from build123d import *

# Parameters (mm, degrees)
BOSS_EXTRUDE1_DEPTH = 1


with BuildPart() as part:
    # Sketch2 → Boss-Extrude1 (new body)
    with BuildSketch(Plane(origin=(0, 0, 0), x_dir=(1, 0, 0), z_dir=(0, 1, 0))):
        with BuildLine():
            Line((-6, 1), (-1, 1))
            Line((-1, 1), (-1, 6))
            ThreePointArc((-1, 6), (-0.853553391, 6.353553391), (-0.5, 6.5))
            Line((-0.5, 6.5), (0.5, 6.5))
            ThreePointArc((0.5, 6.5), (0.853553391, 6.353553391), (1, 6))
            Line((1, 6), (1, 1))
            Line((1, 1), (6, 1))
            ThreePointArc((6, 1), (6.353553391, 0.853553391), (6.5, 0.5))
            Line((6.5, 0.5), (6.5, -0.5))
            ThreePointArc((6.5, -0.5), (6.353553391, -0.853553391), (6, -1))
            Line((6, -1), (1, -1))
            Line((1, -1), (1, -6))
            ThreePointArc((1, -6), (0.853553391, -6.353553391), (0.5, -6.5))
            Line((0.5, -6.5), (-0.5, -6.5))
            ThreePointArc((-0.5, -6.5), (-0.853553391, -6.353553391), (-1, -6))
            Line((-1, -6), (-1, -1))
            Line((-1, -1), (-6, -1))
            ThreePointArc((-6, -1), (-6.353553391, -0.853553391), (-6.5, -0.5))
            Line((-6.5, -0.5), (-6.5, 0.5))
            ThreePointArc((-6.5, 0.5), (-6.353553391, 0.853553391), (-6, 1))
        make_face()
    extrude(amount=BOSS_EXTRUDE1_DEPTH)


solid = part.part
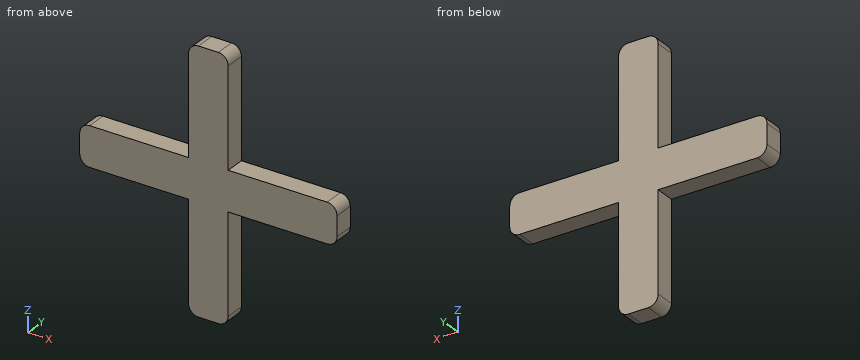
Geometry check sheet. Reference: the model listing, model coordinates, mm. Round coordinates to 2 decimals unless told otherwise and drop trailing zeros. Loops run counter-clockwise (first coordinate to the right, second up) from the corner with the lowest first, then second, coordinate; pieces in that order, holes last. Notation, with made-up numbers: (-38, 88.5) -> (13, 88.5) arc R20 cw to (13, 110.5) -> close; hole circle Ø4 at (11, 18). An arc over 180 degrees is marked (long way). Answer as a JSON object with one key per item and string values. Group by question number.
Item 1: Cross-section at B-B, the plane x = 2.75. Record the cut outline in (y, z).
Item 2: Depth check by flat-ended pin: pin 1 Ø1 at (x, z) = (2.5, -2.5) entering from -Y; pin 2 Ø0.5 at (x, y) = (-4, 0.5) entering from +Z; pin 3 Ø0.5 at (x, y) = (-4, 0.5) entering from -Z; pin 4 Ø2 at (x, z) = (-1.5, 3.5) entering from +Y. Enter the tip coordinate at first touch or a pass-through.
Item 3: Thickness scan on line 1 along X through (y, z) = (0.35, 2); line 2 along Z through (x, y) = (0.75, 0.75). Record the ranges inside material, lowest first.
Item 4: Cross-section at A-A, the plane y = 0.6. Record the cut outline in (x, z).
Item 5: Cross-section at C-C, the plane z = 3.5. Record the cut outline in (x, y), plus the area to 3 significant figures.
Determined:
{
 "1": {"outline": "(0, -1) -> (1, -1) -> (1, 1) -> (0, 1) -> close"},
 "2": {"pin 1": "passes through", "pin 2": "stops at z = 1", "pin 3": "stops at z = -1", "pin 4": "stops at y = 1"},
 "3": {"line 1": "x = -1 to 1", "line 2": "z = -6.43 to 6.43"},
 "4": {"outline": "(-6.5, -0.5) arc R0.5 ccw to (-6, -1) -> (-1, -1) -> (-1, -6) arc R0.5 ccw to (-0.5, -6.5) -> (0.5, -6.5) arc R0.5 ccw to (1, -6) -> (1, -1) -> (6, -1) arc R0.5 ccw to (6.5, -0.5) -> (6.5, 0.5) arc R0.5 ccw to (6, 1) -> (1, 1) -> (1, 6) arc R0.5 ccw to (0.5, 6.5) -> (-0.5, 6.5) arc R0.5 ccw to (-1, 6) -> (-1, 1) -> (-6, 1) arc R0.5 ccw to (-6.5, 0.5) -> close"},
 "5": {"outline": "(-1, 0) -> (1, 0) -> (1, 1) -> (-1, 1) -> close", "area": "2.00 mm²"}
}
